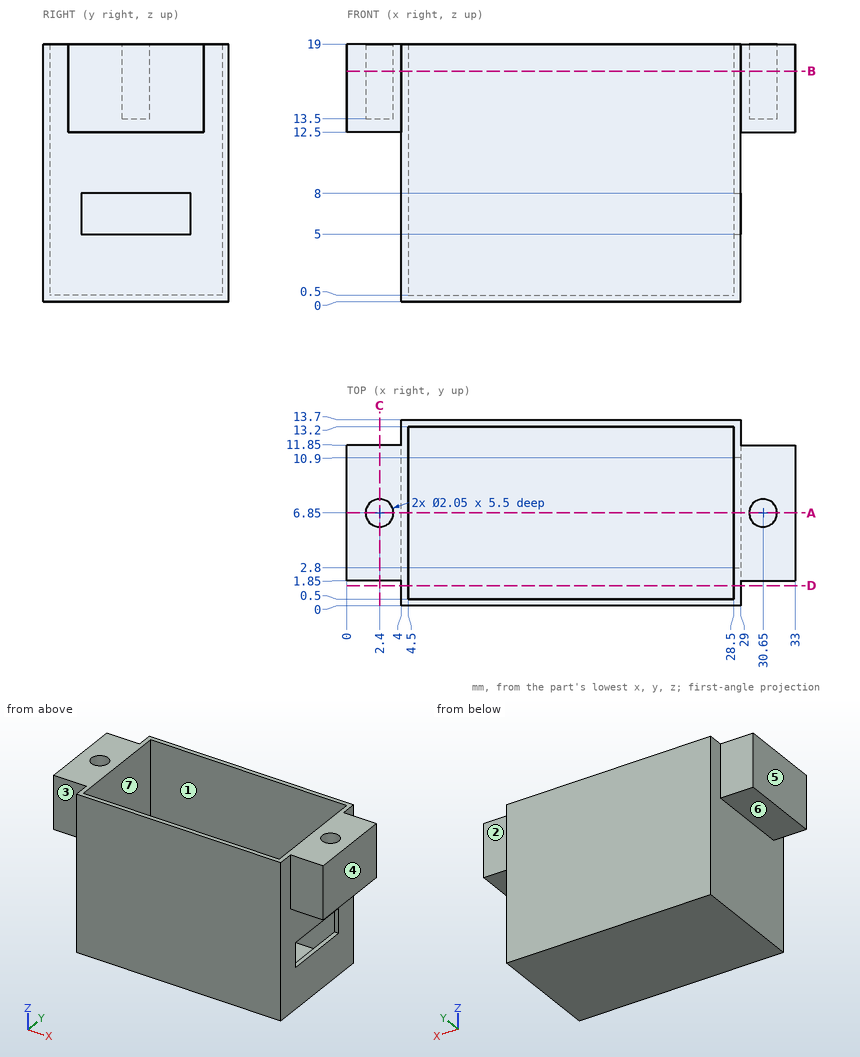
Can you work these out from the drawing? Everything is in mm from the part's minimum corner. A direction names the side the tool comes from. Round coordinates to 2 decimals unless told otherwise and drop trailing zeros. Loops run counter-clockwise (first coordinate to the right, second up) from the corner with the lowest first, then second, coordinate; pieces in that order, holes last. Notation, with made-up numbers: M -37.75,3 L -30.75,3 A33 ccw -30.75,41 Z; hole C 47.5,-5 d9. An arc over 180 degrees is marked long. Write item = value, one per line.
1. I want a section at A-A, the plane y = 6.85. Write out the boundary of the cut face in (x, z) (3 decimals), and give its area (4 significant figures).
Results below:
outline = M 0,12.5 L 4,12.5 L 4,0 L 29,0 L 29,5 L 28.5,5 L 28.5,0.5 L 4.5,0.5 L 4.5,19 L 3.425,19 L 3.425,13.5 L 1.375,13.5 L 1.375,19 L 0,19 Z; M 28.5,8 L 29,8 L 29,12.5 L 33,12.5 L 33,19 L 31.675,19 L 31.675,13.5 L 29.625,13.5 L 29.625,19 L 28.5,19 Z
area = 58.95 mm²
2. Which directions (+Z, -Z, +X, -X, +Y, -Y) give clear straight access to the entire face, cutting with the end or side of a thin tool? Please do the marked faces 1, 2 and 3.
Results below:
face_1 = +Z
face_2 = +Z, -Z, +X, +Y
face_3 = +Z, -Z, -X, -Y
3. I want a section at B-B, the plane z = 17. Write out the boundary of the cut face in (x, y) (3 decimals).
Results below:
outline = M 0,1.85 L 4,1.85 L 4,0 L 29,0 L 29,1.85 L 33,1.85 L 33,11.85 L 29,11.85 L 29,13.7 L 4,13.7 L 4,11.85 L 0,11.85 Z; hole C 2.4,6.85 d2.05; hole M 4.5,0.5 L 28.5,0.5 L 28.5,13.2 L 4.5,13.2 Z; hole C 30.65,6.85 d2.05
4. Will these pins go through, and if not, where does the flat tip stop? P1, Ø2, axis at x = 31.5, y = 5.5, coming from the -Z side; P2, Ø5, axis at y = 2, z = 6, coming from the -X side; P3, Ø1, axis at x = 31, y = 7, coming from the +Z side.
Results below:
P1 = 12.5
P2 = 4
P3 = 13.5
5. Thinking about a two-plate mould opening in X: for the marked faces 4, 5, 6 and 7, which applies, +X half, -X half, draft (parallel to the pull), parting line (faces both ways), or undercut?
Results below:
face_4 = +X half
face_5 = -X half
face_6 = draft
face_7 = undercut
6. I want a section at D-D, the plane y = 1.5. Write out the boundary of the cut face in (x, z).
Results below:
outline = M 4,0 L 29,0 L 29,19 L 28.5,19 L 28.5,0.5 L 4.5,0.5 L 4.5,19 L 4,19 Z
7. I want a section at C-C, the plane x = 2.4. Write out the boundary of the cut face in (y, z) (3 decimals).
Results below:
outline = M 1.85,12.5 L 11.85,12.5 L 11.85,19 L 7.875,19 L 7.875,13.5 L 5.825,13.5 L 5.825,19 L 1.85,19 Z
8. I need wall thicknesses on probe 1 along X at (y, z) = (5.25, 4.5); probe 2 along Y at (x, z) = (5.5, 14.25); probe 3 along X at (y, z) = (7.5, 18). Which ranges of each line are inside material? Lowest first, please.
Results below:
probe_1 = 4 to 4.5, 28.5 to 29
probe_2 = 0 to 0.5, 13.2 to 13.7
probe_3 = 0 to 1.61, 3.19 to 4.5, 28.5 to 29.86, 31.44 to 33
